Design review of the part built by this model. Coordinates are the model's own, in mm. A direction names the side the tool comes from. Coordinates: 2 decimals unless noted, no trailing zeros. Write each loop counter-clockwise with the first axis right and the second up, starting at its lowest first coordinate (ties: lowest second). Pieces come first, ordered by that corner, then holes. Notation, with made-up numbers: (8.5, -18) - (61.5, -18) arc R21 ccw to (61.5, -11) - close; hole circle Ø11 at (-4.5, 8.25). An arc over 180 degrees is marked (long way). Answer as a JSON object with one key per item and string values.
```python
from build123d import *

# Parameters (mm, degrees)
SKETCH2_R           = 0.500109693
BOSS_EXTRUDE1_DEPTH = 5
BOSS_EXTRUDE2_DEPTH = 1


with BuildPart() as part:
    # Sketch2 → Boss-Extrude1 (new body)
    with BuildSketch(Plane(origin=(0, 0, 0), x_dir=(1, 0, 0), z_dir=(0, 0, -1))):
        with BuildLine():
            Line((29.97295835, 6.642737104), (28.862437793, 5.215722686))
            Line((28.862437793, 5.215722686), (29.97295835, 3.953817374))
            add(Edge.make_bspline(
                [(5.565346412, 3.953817374), (17.919076804, -3.939717318), (29.97295835, 3.953817374)],
                knots=[0, 0, 0, 1, 1, 1], degree=2))
            Line((5.565346412, 3.953817374), (0, 0.570103483))
            Line((0, 0.570103483), (2.65645961, 5.215722686))
            Line((2.65645961, 5.215722686), (0, 9.556126627))
            Line((0, 9.556126627), (5.565346412, 6.285726684))
            add(Edge.make_bspline(
                [(5.565346412, 6.285726684), (12.037313538, 11.217277608), (22.14175538, 12.07873787), (29.97295835, 6.642737104)],
                knots=[0, 0, 0, 0, 1, 1, 1, 1], degree=3))
        make_face()
        with Locations(Location((26.5225963, 6.780666166, 0), (0, 0, 180))):
            Circle(SKETCH2_R, mode=Mode.SUBTRACT)
    extrude(amount=-BOSS_EXTRUDE1_DEPTH)

    # Sketch4 → Boss-Extrude2 (add)
    with BuildSketch(Plane(origin=(0, 0, 5), x_dir=(-1, 0, 0), z_dir=(0, 0, 1))):
        with BuildLine():
            Line((-17.330711562, 1.879075557), (-19.398244519, 1.879075557))
            add(Edge.make_bspline(
                [(-19.398244519, 1.879075557), (-19.857893705, 3.836469275), (-21.838627479, 5.07519839)],
                knots=[0, 0, 0, 1, 1, 1], degree=2))
            Line((-21.838627479, 5.07519839), (-21.838627479, 7.118264722))
            Line((-21.838627479, 7.118264722), (-12.493271281, 7.118264722))
            Line((-12.493271281, 7.118264722), (-12.493271281, 4.559250574))
            Line((-12.493271281, 4.559250574), (-18.4990791, 4.559250574))
            add(Edge.make_bspline(
                [(-18.4990791, 4.559250574), (-18.040909727, 3.659817697), (-17.443363766, 2.880283759), (-17.330711562, 1.879075557)],
                knots=[0, 0, 0, 0, 1, 1, 1, 1], degree=3))
        make_face()
    extrude(amount=BOSS_EXTRUDE2_DEPTH)


solid = part.part
```
(1) Take a section at B-B, the plane x = 4.5. Write out the cut boundary in (y, z).
Solved:
{"outline": "(-6.91, 0) - (-3.31, 0) - (-3.31, 5) - (-6.91, 5) - close"}
(2) The part is to be moulded in two halves that separate along X. For faces 6 (the face through (2.822, -2.286, 2.465)), 7 (the face through (21.839, -6.1, 5.5)), 8 (the face through (2.744, -7.944, 2.465)), 9 (the face through (17.2, -7.118, 5.5)), say which applies: pulls with the +X half, pulls with the -X half, needs draft (parallel to the pull), parting line crosses it, or undercut.
Solved:
{"face 6": "undercut", "face 7": "pulls with the +X half", "face 8": "undercut", "face 9": "needs draft"}
(3) To check wall thickness, follow line 1 (X direction, y = -6.75, z = 2.5); line 2 (X direction, y = -7, z = 3.5); line 3 (Z direction, x = 26, y = -5.25). State the ranges of each line that lie inside material, in increasing order. Write a range as from..to.
Solved:
{"line 1": "x = 1.72..4.78, 6.2..26.02, 27.02..29.82", "line 2": "x = 1.56..4.35, 6.57..26.07, 26.97..29.44", "line 3": "z = 0..5"}
(4) Take a section at A-A, the plane y = -5.5. Write out the cut boundary in (x, z), and give its area (3 significant figures).
Solved:
{"outline": "(2.48, 0) - (29.08, 0) - (29.08, 5) - (21.84, 5) - (21.84, 6) - (12.49, 6) - (12.49, 5) - (2.48, 5) - close", "area": "142 mm^2"}
(5) For pin 1 (2 mm diameter, centred on y = -1.5, z = 3, fed in from -X); pin 2 (1 mm diameter, centred on y = -2.5, z = 2.5, fed in from -X); pin 3 (4 mm diameter, centred on x = 4, y = -2.5, fed in from +Z), all flat-tipped, find the tip position at first contact; note any pin that passes through.
Solved:
{"pin 1": "stops at x = 0", "pin 2": "stops at x = 0.82", "pin 3": "stops at z = 5"}
(6) Tool access review of faces 1 (the face through (15.5, -4.559, 5.5)), 2 (the face through (18.4, -1.879, 5.5)), 3 (the face through (29.425, -5.939, 2.465)), 4 (the face through (12.493, -5.9, 5.5)), 5 (the face through (1.31, -2.86, 2.46)): name each direction out of +Z, -Z, +X, -X, +Y, -Y from which nothing blocks a thin tool from reaching the whole face with its end or side.
Solved:
{"face 1": "+Z, -X", "face 2": "+Z, +X, -X, +Y", "face 3": "+Z, -Z, +X", "face 4": "+Z, -X, +Y, -Y", "face 5": "+Z, -Z, -X"}
